from build123d import *

# Parameters (mm, degrees)
F0_R     = 2.5853808969
F1_DEPTH = 3.78621
F2_W     = 92.5128534436
F2_H     = 67.3747956753
F2_W_2   = 88.2868915796
F2_H_2   = 63.4562075138
F3_DEPTH = 25.4
F4_W     = 92.5128534436
F4_H     = 67.3747956753
F5_DEPTH = 5.39071


with BuildPart() as f1:
    # F0 (on Top) → F1 (new body)
    with BuildSketch(Plane.XY):
        with Locations((-6.1489455687, 15.4150508655)):
            Circle(F0_R)
        with Locations((-38.6942066252, 26.1586811393)):
            Circle(F0_R)
        with Locations((-22.1503593461, 26.1586811393)):
            Circle(F0_R)
        with Locations((10.1477103229, -15.5244964796)):
            Circle(F0_R)
        with Locations((-30.1908456923, -25.8376869994)):
            Circle(F0_R)
        with Locations((-22.1749195264, -15.5244964796)):
            Circle(F0_R)
        with Locations((25.4185836632, 26.1586811393)):
            Circle(F0_R)
        with Locations((25.3940272081, 15.4150508655)):
            Circle(F0_R)
        with Locations((10.1477084602, -5.211315273)):
            Circle(F0_R)
        with Locations((-30.4178264261, 26.1586811393)):
            Circle(F0_R)
        with Locations((17.6428148795, -15.5244964796)):
            Circle(F0_R)
        with Locations((25.3940216202, -5.211315273)):
            Circle(F0_R)
        with Locations((10.1477140482, 15.4150508655)):
            Circle(F0_R)
        with Locations((-22.1749158012, 15.4150508655)):
            Circle(F0_R)
        with Locations((-14.4147922161, 15.4150508655)):
            Circle(F0_R)
        with Locations((17.6428186047, 15.4150508655)):
            Circle(F0_R)
        with Locations((17.6428130168, -5.211315273)):
            Circle(F0_R)
        with Locations((-22.1749213891, -5.211315273)):
            Circle(F0_R)
        with Locations((32.1207015841, 15.4150508655)):
            Circle(F0_R)
        with Locations((-21.9233786123, -25.8376869994)):
            Circle(F0_R)
        with Locations((25.3940234828, -15.5244964796)):
            Circle(F0_R)
        with Locations((-38.7187686683, -5.211315273)):
            Circle(F0_R)
        with Locations((-30.4423907975, 5.1018668649)):
            Circle(F0_R)
        with Locations((39.3573794852, -15.5244964796)):
            Circle(F0_R)
        with Locations((39.3819396656, 26.1586811393)):
            Circle(F0_R)
        with Locations((-30.4423866065, -15.5244964796)):
            Circle(F0_R)
        with Locations((17.6673750598, 26.1586811393)):
            Circle(F0_R)
        with Locations((-14.390235761, 26.1586811393)):
            Circle(F0_R)
        with Locations((2.7696161597, -25.8376869994)):
            Circle(F0_R)
        with Locations((-5.8974083799, -25.8376869994)):
            Circle(F0_R)
        with Locations((2.5180789708, 15.4150508655)):
            Circle(F0_R)
        with Locations((-6.1489511567, -5.211315273)):
            Circle(F0_R)
        with Locations((32.1206936679, 5.1018668649)):
            Circle(F0_R)
        with Locations((-22.1749237174, 5.1018668649)):
            Circle(F0_R)
        with Locations((-38.7187630803, 15.4150508655)):
            Circle(F0_R)
        with Locations((-14.1632550272, -25.8376869994)):
            Circle(F0_R)
        with Locations((2.5426354259, 26.1586811393)):
            Circle(F0_R)
        with Locations((-6.1243891136, 26.1586811393)):
            Circle(F0_R)
        with Locations((32.1452580392, 26.1586811393)):
            Circle(F0_R)
        with Locations((10.1722705033, 26.1586811393)):
            Circle(F0_R)
        with Locations((-38.7187709966, 5.1018668649)):
            Circle(F0_R)
        with Locations((39.3573752943, 5.1018668649)):
            Circle(F0_R)
        with Locations((2.5180733829, -5.211315273)):
            Circle(F0_R)
        with Locations((17.8943557936, -25.8376869994)):
            Circle(F0_R)
        with Locations((-14.4148001324, 5.1018668649)):
            Circle(F0_R)
        with Locations((-38.4672258914, -25.8376869994)):
            Circle(F0_R)
        with Locations((2.5180710546, 5.1018668649)):
            Circle(F0_R)
        with Locations((32.372238773, -25.8376869994)):
            Circle(F0_R)
        with Locations((39.3573832105, 15.4150508655)):
            Circle(F0_R)
        with Locations((39.3573776226, -5.211315273)):
            Circle(F0_R)
        with Locations((-30.4423828812, 15.4150508655)):
            Circle(F0_R)
        with Locations((2.5180752455, -15.5244964796)):
            Circle(F0_R)
        with Locations((10.1477061319, 5.1018668649)):
            Circle(F0_R)
        with Locations((-30.4423884691, -5.211315273)):
            Circle(F0_R)
        with Locations((39.6089203994, -25.8376869994)):
            Circle(F0_R)
        with Locations((-6.148953485, 5.1018668649)):
            Circle(F0_R)
        with Locations((32.1206978588, -15.5244964796)):
            Circle(F0_R)
        with Locations((-14.4147959414, -15.5244964796)):
            Circle(F0_R)
        with Locations((25.645564397, -25.8376869994)):
            Circle(F0_R)
        with Locations((25.3940192918, 5.1018668649)):
            Circle(F0_R)
        with Locations((-38.7187668056, -15.5244964796)):
            Circle(F0_R)
        with Locations((-6.148949294, -15.5244964796)):
            Circle(F0_R)
        with Locations((10.399251237, -25.8376869994)):
            Circle(F0_R)
        with Locations((17.6428106885, 5.1018668649)):
            Circle(F0_R)
        with Locations((32.1206959962, -5.211315273)):
            Circle(F0_R)
        with Locations((-14.4147978041, -5.211315273)):
            Circle(F0_R)
    extrude(amount=F1_DEPTH)



with BuildPart() as f3:
    # F2 (on Top) → F3 (new body)
    with BuildSketch(Plane.XY):
        Rectangle(F2_W, F2_H)
        Rectangle(F2_W_2, F2_H_2, mode=Mode.SUBTRACT)
    extrude(amount=F3_DEPTH)


with BuildPart() as f1_1:
    add(f1.part)

    add(f3.part)  # F5 merges F3
    # F4 (on face) → F5 (join)
    with BuildSketch(Plane(origin=(0, 0, 0), x_dir=(1, 0, 0), z_dir=(0, 0, -1))):
        Rectangle(F4_W, F4_H)
    extrude(amount=F5_DEPTH)


solid = f1_1.part
For this review, take the finished solid that the model builds, in its own axes (mm). Round coordinates to 2 decimals unless told otherwise and drop trailing zeros. Order: outer loops, then holes, each group sorted by start corner. A loop starts at its lowest first (then second) coordinate and runs counter-clockwise, first axis right, second up. Notation, with made-up numbers: M 1,32.25 L 16,32.25 A12 ccw 16,51.25 Z; hole C 88.25,-2 d7. An arc over 180 degrees is marked long. Use a Markdown table: item, result. Add a question column.
Item 1: Add section B-B, the plane z = 11. Give the boundary of the cut face in (x, y), then the cut area to 3 significant figures.
Item 2: Mouldability with a two-part tool opening along Y and no side actions: class faces 1 (the cylindrical face through (8.24, 17.16, 1.87)), 2 (the flat face through (-1, 33.687, 10)), 3 (the cylindrical face through (41.82, -4.43, 1.87)) as released by +Y, released by -Y, zero draft, split by the parting line, or undercut.
Item 3: To check wall thickness, follow line 1 along X through (y, z) = (6.5, 5.5); line 2 along Y through (x, z) = (-26, 23.5); line 3 along Z through (x, y) = (-10, -19). State the ranges of each line that lie inside material, in increasing order.
Item 4: Add section A-A, the plane y = -10. Give the boundary of the cut face in (x, z), then the cut area to 3 significant figures.
Item 5: Add section D-D, the plane z = 2.5. State how many separate pieces and enclosed holes the cut face has, then the cut area to 3 significant figures.
Item 6: Insertion check: pin 1 (1.6 mm diameter, centred on x = 26.5, y = -15, fed in from +Z). The pin has a flat end and moves straight along its axis. Give the tip position at first contact, or say it passes through.
Geometry results:
| question | item | result |
|---|---|---|
| 1 | outline | M -46.26,-33.69 L 46.26,-33.69 L 46.26,33.69 L -46.26,33.69 Z; hole M -44.14,-31.73 L 44.14,-31.73 L 44.14,31.73 L -44.14,31.73 Z |
| 1 | area | 631 mm² |
| 2 | face 1 | undercut |
| 2 | face 2 | released by +Y |
| 2 | face 3 | undercut |
| 3 | line 1 | x = -46.26 to -44.14, 44.14 to 46.26 |
| 3 | line 2 | y = -33.69 to -31.73, 31.73 to 33.69 |
| 3 | line 3 | z = -5.39 to 0 |
| 4 | outline | M -46.26,-5.39 L 46.26,-5.39 L 46.26,25.4 L 44.14,25.4 L 44.14,0 L -44.14,0 L -44.14,25.4 L -46.26,25.4 Z |
| 4 | area | 606 mm² |
| 5 | separate pieces | 67 |
| 5 | enclosed holes | 1 |
| 5 | area | 2,020 mm² |
| 6 | pin 1 | stops at z = 3.79 |
